Autodesk Inventor part; units mm, degrees
ref_plane "YZ Plane" through (0, 0, 0) normal (1, 0, 0) x (0, 1, 0)
ref_plane "XZ Plane" through (0, 0, 0) normal (0, 1, 0) x (-1, 0, 0)
ref_plane "XY Plane" through (0, 0, 0) normal (0, 0, 1) x (1, 0, 0)
sketch "Sketch1" plane through (0, 0, 0) normal (0, 1, 0) x (-1, 0, 0)
  circle A0 centre (0, 0) radius 12.7
  circle A1 centre (0, 0) radius 11
  dimension "d0" = 25.4
  dimension "d1" = 22
extrude "Extrusion1" add sketch "Sketch1" along normal blind 300
sketch "Sketch2" plane through (0, 0, 0) normal (1, 0, 0) x (0, 1, 0)
  circle A0 centre (100, 0) radius 3
  line L0 (0, -12.7) -> (0, 12.7)
  circle A1 centre (15, 0) radius 2.5
  point P0 (0, 0)
  dimension "d4" = 6
  dimension "d5" = 100
  dimension "d6" = 5
  dimension "d7" = 15
extrude "Extrusion2" cut sketch "Sketch2" along normal mid plane 300
properties part number "stickshift"
For this review, take the finished solid that the model builds, in its own axes (mm). Round coordinates to 2 decimals unless told otherwise and drop trailing zeros. Write each loop counter-clockwise with the first axis right and the second up, starting at its lowest first coordinate (ties: lowest second). Pieces come first, ordered by that corner, then holes. Notation, with made-up numbers: (85.5, -18) - (142.5, -18) arc R30 ccw to (142.5, 6) - close; hole circle Ø9 at (80, -7.75). An arc over 180 degrees is marked (long way). Use CSV: the item, a comma, the result in double quotes.
1) Wall thickness on line 1 along Y through (x, z) = (-12.05, 0); line 2 along Z through (x, y) = (-0.5, 128.5); line 3 along X through (y, z) = (86.5, 0): over which ranges is each line inside the solid? List them lowest first. Write a range as from..to.
Conclusion:
line 1,"y = 0..12.5, 17.5..97, 103..300"
line 2,"z = -12.69..-10.99, 10.99..12.69"
line 3,"x = -12.7..-11, 11..12.7"
2) Clearance check with flat-ended pins moving along their axes: pin 1 Ø8 at (y, z) = (120, 5.5) entering from +X; pin 2 Ø4.5 at (y, z) = (15, 0) entering from +X; pin 3 Ø5 at (y, z) = (34.5, -9) entering from -X; pin 4 Ø8 at (y, z) = (164.5, 7) entering from +X. State where each tip first meets the part, or that it passes through.
Conclusion:
pin 1,"stops at x = 12.61"
pin 2,"passes through"
pin 3,"stops at x = -10.91"
pin 4,"stops at x = 12.34"
3) Add section C-C on y = 15. Write out the cut boundary in (x, z), and give its area (3 significant figures).
Conclusion:
outline,"(-12.45, -2.5) arc R12.7 ccw to (12.45, -2.5) - (10.71, -2.5) arc R11 cw to (-10.71, -2.5) - close; (-12.45, 2.5) - (-10.71, 2.5) arc R11 cw to (10.71, 2.5) - (12.45, 2.5) arc R12.7 ccw to start"
area,"109 mm^2"
4) The part is to be moulded in two halves that separate along Y. For faces 1 (the cylindrical face through (-10.161, 147.9, 4.213)), 2 (the flat face through (0.1, 0, 11.3)), 3 (the cylindrical face through (-11.63, 99.35, -2.93)), say which applies: pulls with the +Y half, pulls with the -Y half, needs draft (parallel to the pull), parting line crosses it, or undercut.
Conclusion:
face 1,"needs draft"
face 2,"pulls with the -Y half"
face 3,"undercut"
5) Add section D-D on y = 82. Write out the cut boundary in (x, z), and give its area (3 significant figures).
Conclusion:
outline,"circle Ø25.4 at (0, 0); hole circle Ø22 at (0, 0)"
area,"127 mm^2"
6) Add section B-B on x = 0. Write out the cut boundary in (y, z).
Conclusion:
outline,"(0, -12.7) - (300, -12.7) - (300, -11) - (0, -11) - close; (0, 11) - (300, 11) - (300, 12.7) - (0, 12.7) - close"
7) Add section A-A on z = 0. Write out the cut boundary in (x, y).
Conclusion:
outline,"(-12.7, 0) - (-11, 0) - (-11, 12.5) - (-12.7, 12.5) - close; (-12.7, 17.5) - (-11, 17.5) - (-11, 97) - (-12.7, 97) - close; (-12.7, 103) - (-11, 103) - (-11, 300) - (-12.7, 300) - close; (11, 0) - (12.7, 0) - (12.7, 12.5) - (11, 12.5) - close; (11, 17.5) - (12.7, 17.5) - (12.7, 97) - (11, 97) - close; (11, 103) - (12.7, 103) - (12.7, 300) - (11, 300) - close"
